from build123d import *

# Parameters (mm, degrees)
SKETCH1_R           = 5.7
SKETCH1_R_2         = 2.55
BOSS_EXTRUDE1_DEPTH = 12
SKETCH2_R           = 1.65
BOSS_EXTRUDE2_DEPTH = 6


with BuildPart() as part:
    # Sketch1 → Boss-Extrude1 (new body)
    with BuildSketch(Plane(origin=(0, 0, 0), x_dir=(1, 0, 0), z_dir=(0, 1, 0))):
        with Locations(Location((0, 0, 0), (0, 0, 270))):
            Circle(SKETCH1_R)
        with Locations(Location((0, 0, 0), (0, 0, 270))):
            Circle(SKETCH1_R_2, mode=Mode.SUBTRACT)
    extrude(amount=BOSS_EXTRUDE1_DEPTH)

    # Sketch2 → Boss-Extrude2 (add)
    with BuildSketch(Plane(origin=(0, 12, 0), x_dir=(1, 0, 0), z_dir=(0, 1, 0))):
        Polygon((6.92820323, 0), (3.464101615, 6), (-3.464101615, 6), (-6.92820323, 0), (-3.464101615, -6), (3.464101615, -6), align=None)
        with Locations(Location((0, 0, 0), (0, 0, 270))):
            Circle(SKETCH2_R, mode=Mode.SUBTRACT)
    extrude(amount=BOSS_EXTRUDE2_DEPTH)


solid = part.part
Verification items for the finished model (mm, model axes). A direction names the side the tool comes from. Give positions to 0.01 mm unless a question says otherwise; leave off trailing zeros. Write each loop counter-clockwise with the first axis right and the second up, starting at its lowest first coordinate (ties: lowest second). Pieces come first, ordered by that corner, then holes.
(1) Gauge pin test, flat ends, axial feed: pin 1 (5 mm diameter, centred on y = 15.5, z = 2, fed in from +X); pin 2 (6 mm diameter, centred on y = 2.5, z = 4, fed in from -X); pin 3 (1.5 mm diameter, centred on y = 3, z = 2, fed in from +X). Record the tip position at first contact, or that the pin passes through.
(2) Cross-section at B-B (y = 15.75). Enter the section's corners in (x, z).
(3) Cross-section at D-D (x = -2). Enter the section's corners in (y, z).
(4) Cross-section at C-C (z = 3.25). Enter the section's corners in (x, y).
(5) Cross-section at A-A (x = 0). Enter the section's corners in (y, z).
(6) Mould release check, pull along X, two halves, no side actions. Record for faces 3 (the face through (-2.5, 0, 1.2)), 4 (the face through (0.77, 5.92, 2.43)), 5 (the face through (-5.22, 14.96, 2.96)): +X half, -X half, draft (parallel to the pull), parting line (faces both ways), or undercut.
(7) Access from +Z, -Z, +X, -X, +Y, -Y to the whole of each face (thin tool, end or side, straight path). Record for faces 1 (the face through (-3.5, 5.9, -4.5)), 2 (the face through (0, 15, -6)).
(8) Material ranges on line 1 (X direction, y = 5.75, z = 0); line 2 (X direction, y = 11.25, z = 2); line 3 (Z direction, x = 0.5, y = 4.5), recorded low to high.
Worked out:
1. pin 1: stops at x = 6.93
1. pin 2: stops at x = -5.61
1. pin 3: stops at x = 5.56
2. outline: (-6.93, 0) - (-3.46, -6) - (3.46, -6) - (6.93, 0) - (3.46, 6) - (-3.46, 6) - close; hole circle Ø3.3 at (0, 0)
3. outline: (0, -5.34) - (12, -5.34) - (12, -6) - (18, -6) - (18, 6) - (12, 6) - (12, 5.34) - (0, 5.34) - (0, 1.58) - (12, 1.58) - (12, -1.58) - (0, -1.58) - close
4. outline: (-5.05, 12) - (-4.68, 12) - (-4.68, 0) - (4.68, 0) - (4.68, 12) - (5.05, 12) - (5.05, 18) - (-5.05, 18) - close
5. outline: (0, -5.7) - (12, -5.7) - (12, -6) - (18, -6) - (18, -1.65) - (12, -1.65) - (12, -2.55) - (0, -2.55) - close; (0, 2.55) - (12, 2.55) - (12, 1.65) - (18, 1.65) - (18, 6) - (12, 6) - (12, 5.7) - (0, 5.7) - close
6. face 3: draft
6. face 4: undercut
6. face 5: -X half
7. face 1: -Y
7. face 2: -Z, +X, -X, +Y, -Y
8. line 1: x = -5.7 to -2.55, 2.55 to 5.7
8. line 2: x = -5.34 to -1.58, 1.58 to 5.34
8. line 3: z = -5.68 to -2.5, 2.5 to 5.68
